Autodesk Inventor part; units mm, degrees
ref_plane "YZ Plane" through (0, 0, 0) normal (1, 0, 0) x (0, 1, 0)
ref_plane "XZ Plane" through (0, 0, 0) normal (0, 1, 0) x (-1, 0, 0)
ref_plane "XY Plane" through (0, 0, 0) normal (0, 0, 1) x (1, 0, 0)
sketch "Sketch1" plane through (0, 0, 0) normal (0, 1, 0) x (-1, 0, 0)
  line L0 (0, 0) -> (203.2, 0)
  line L1 (203.2, 0) -> (203.2, -279.4)
  line L2 (203.2, -279.4) -> (0, -279.4)
  line L3 (0, -279.4) -> (0, 0)
  dimension "d0" = 203.2
  dimension "d1" = 279.4
extrude "Plate1" add sketch "Sketch1" along normal blind 3.048
sketch "Sketch2" plane through (0, 3.048, 0) normal (0, 1, 0) x (1, 0, 0)
  circle A0 centre (-12.7, 12.7) radius 2.5019
  line L0 (0, 0) -> (-203.2, 0)
  line L1 (0, 279.4) -> (0, 0)
  circle A1 centre (-25.4, 12.7) radius 2.5019
  circle A2 centre (-38.1, 12.7) radius 2.5019
  circle A3 centre (-50.8, 12.7) radius 2.5019
  circle A4 centre (-63.5, 12.7) radius 2.5019
  circle A5 centre (-76.2, 12.7) radius 2.5019
  circle A6 centre (-88.9, 12.7) radius 2.5019
  circle A7 centre (-101.6, 12.7) radius 2.5019
  circle A8 centre (-114.3, 12.7) radius 2.5019
  circle A9 centre (-127, 12.7) radius 2.5019
  circle A10 centre (-139.7, 12.7) radius 2.5019
  circle A11 centre (-152.4, 12.7) radius 2.5019
  circle A12 centre (-165.1, 12.7) radius 2.5019
  circle A13 centre (-177.8, 12.7) radius 2.5019
  circle A14 centre (-190.5, 12.7) radius 2.5019
  line L2 (-203.2, 0) -> (-203.2, 279.4)
  circle A15 centre (-190.5, 25.4) radius 2.5019
  circle A16 centre (-190.5, 38.1) radius 2.5019
  circle A17 centre (-190.5, 50.8) radius 2.5019
  circle A18 centre (-190.5, 63.5) radius 2.5019
  circle A19 centre (-190.5, 76.2) radius 2.5019
  circle A20 centre (-190.5, 88.9) radius 2.5019
  circle A21 centre (-190.5, 101.6) radius 2.5019
  circle A22 centre (-190.5, 114.3) radius 2.5019
  circle A23 centre (-190.5, 127) radius 2.5019
  circle A24 centre (-190.5, 139.7) radius 2.5019
  circle A25 centre (-190.5, 152.4) radius 2.5019
  circle A26 centre (-190.5, 165.1) radius 2.5019
  circle A27 centre (-190.5, 177.8) radius 2.5019
  circle A28 centre (-190.5, 190.5) radius 2.5019
  circle A29 centre (-190.5, 203.2) radius 2.5019
  circle A30 centre (-190.5, 215.9) radius 2.5019
  circle A31 centre (-190.5, 228.6) radius 2.5019
  circle A32 centre (-190.5, 241.3) radius 2.5019
  circle A33 centre (-190.5, 254) radius 2.5019
  circle A34 centre (-190.5, 266.7) radius 2.5019
  line L3 (-203.2, 279.4) -> (0, 279.4)
  circle A35 centre (-177.8, 266.7) radius 2.5019
  circle A36 centre (-165.1, 266.7) radius 2.5019
  circle A37 centre (-152.4, 266.7) radius 2.5019
  circle A38 centre (-139.7, 266.7) radius 2.5019
  circle A39 centre (-127, 266.7) radius 2.5019
  circle A40 centre (-114.3, 266.7) radius 2.5019
  circle A41 centre (-101.6, 266.7) radius 2.5019
  circle A42 centre (-88.9, 266.7) radius 2.5019
  circle A43 centre (-76.2, 266.7) radius 2.5019
  circle A44 centre (-63.5, 266.7) radius 2.5019
  circle A45 centre (-50.8, 266.7) radius 2.5019
  circle A46 centre (-38.1, 266.7) radius 2.5019
  circle A47 centre (-25.4, 266.7) radius 2.5019
  circle A48 centre (-12.7, 266.7) radius 2.5019
  circle A49 centre (-12.7, 254) radius 2.5019
  circle A50 centre (-12.7, 241.3) radius 2.5019
  circle A51 centre (-12.7, 228.6) radius 2.5019
  circle A52 centre (-12.7, 215.9) radius 2.5019
  circle A53 centre (-12.7, 203.2) radius 2.5019
  circle A54 centre (-12.7, 190.5) radius 2.5019
  circle A55 centre (-12.7, 177.8) radius 2.5019
  circle A56 centre (-12.7, 165.1) radius 2.5019
  circle A57 centre (-12.7, 152.4) radius 2.5019
  circle A58 centre (-12.7, 139.7) radius 2.5019
  circle A59 centre (-12.7, 127) radius 2.5019
  circle A60 centre (-12.7, 114.3) radius 2.5019
  circle A61 centre (-12.7, 101.6) radius 2.5019
  circle A62 centre (-12.7, 88.9) radius 2.5019
  circle A63 centre (-12.7, 76.2) radius 2.5019
  circle A64 centre (-12.7, 63.5) radius 2.5019
  circle A65 centre (-12.7, 50.8) radius 2.5019
  circle A66 centre (-12.7, 38.1) radius 2.5019
  circle A67 centre (-12.7, 25.4) radius 2.5019
  dimension "d3" = 5.0038
  dimension "d4" = 12.7
  dimension "d5" = 12.7
  dimension "d8" = 12.7
  dimension "d13" = 5.0038
  dimension "d15" = 12.7
  dimension "d16" = 12.7
  dimension "d19" = 12.7
  dimension "d24" = 5.0038
  dimension "d25" = 12.7
  dimension "d26" = 12.7
  dimension "d29" = 12.7
  dimension "d34" = 5.0038
  dimension "d35" = 12.7
  dimension "d36" = 12.7
  dimension "d39" = 12.7
extrude "Extrusion1" cut sketch "Sketch2" against normal blind 25.4 contours A0 | A1 | A2 | A3 | A4 | A5 | A6 | A7 | A8 | A9 | A10 | A11 | A12 | A13 | A14 | A15 | A16 | A17 | A18 | A19 | A20 | A21 | A22 | A23 | A24 | A25 | A26 | A27 | A28 | A29 | A30 | A31 | A32 | A33 | A34 | A35 | A36 | A37 | A38 | A39 | A40 | A41 | A42 | A43 | A44 | A45 | A46 | A47 | A48 | A49 | A50 | A51 | A52 | A53 | A54 | A55 | A56 | A57 | A58 | A59 | A60 | A61 | A62 | A63 | A64 | A65 | A66 | A67
equation "\"d2\" = Thickness"
equation "\"BendRadius\" = Thickness"
equation "\"BendReliefWidth\" = Thickness"
equation "\"BendReliefDepth\" = 0.5 * Thickness"
equation "\"CornerReliefSize\" = 4 * Thickness"
equation "\"MinimumRemnant\" = 2 * Thickness"
equation "\"TransitionRadius\" = BendRadius"
equation "\"JacobiRadiusSize\" = BendRadius"
equation "\"GapSize\" = Thickness"
properties part number "Bottom Plate"
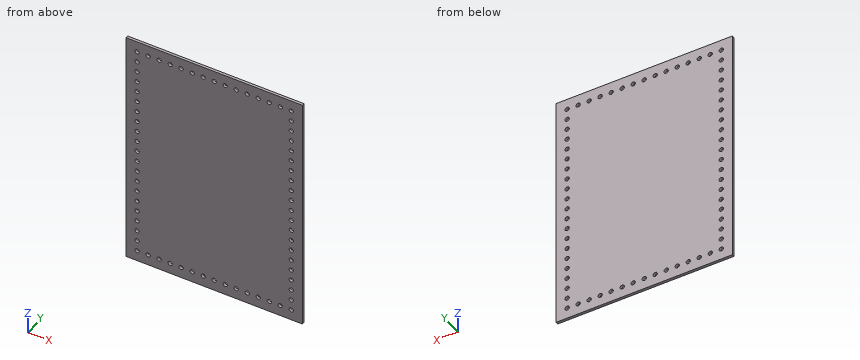
CAD build for the part. Positions are in the model's coordinates, mm. Round coordinates to 2 decimals unless told otherwise and drop trailing zeros. Put each result on its own line as item: value. Start each with the question number.
1) Pin check, flat tip, straight feed: pin 1 Ø3 at (x, z) = (-12.7, -177.8) entering from +Y. Stop position of the tip, or through.
2) Drill centre lines: probe 1 along X at (y, z) = (1.1, -139.7); probe 2 along X at (y, z) = (0.4, -26); probe 3 along Z at (x, y) = (-52, 2.15). Where is each one in solid material? Low to high. Write a range as [from, to].
3) Saw through at A-A, the plane y = 0.6. Count the separate pieces of the cut face and the enclosed holes in it, and give its area (3 significant figures).
Resolved:
1. pin 1: through
2. probe 1: [-203.2, -193], [-188, -15.2], [-10.2, 0]
2. probe 2: [-203.2, -192.93], [-188.07, -15.13], [-10.27, 0]
2. probe 3: [-279.4, -268.9], [-264.5, -14.9], [-10.5, 0]
3. separate pieces: 1
3. enclosed holes: 68
3. area: 55,400 mm²
